Geometry: final body of the model. Coordinates: model frame, mm. A direction names the side the tool comes from. Give positions to 0.01 mm unless a question says otherwise; leave off trailing zeros. Write each loop counter-clockwise with the first axis right and the second up, starting at its lowest first coordinate (ties: lowest second). Pieces come first, ordered by that corner, then holes. Notation, with made-up numbers: M 0.5,13.5 L 36.5,13.5 A17 cw 36.5,24.5 Z; hole C 80.25,-12 d9. An arc over 180 degrees is marked long. Use one line per item in the form item = value. Start each with the question number.
Item 1: Material intervals for line 1 along Y through (x, z) = (37, 4.6); line 2 along X through (y, z) = (-3, 4.8); line 3 along X through (y, z) = (27, 3.95), sorted ascending. Write a range as from..to.
Item 2: Access query for faces 4 (the flat face through (-24.4, 4.5, 4.6)), 5 (the flat face through (63, 1, 5.08)). Directions: +Z, -Z, +X, -X, +Y, -Y. A direction counts if a zero-diameter tool reaches every point of the face in a straight line with its end or side. Return the directions, or none.
Item 3: Contact query for flat-ended pins moving along their axis: P1, Ø2, axis at x = 31, z = 4.5, coming from the -Y side; P2, Ø0.8, axis at x = 57, y = 29.5, coming from the -Z side; P3, Ø2, axis at x = 91.5, y = 29.5, coming from the +Z side; P4, Ø1.4, axis at x = 28, z = 1.5, coming from the +Y side. Output: stop coordinate, or through.
Item 4: Pull-direction query (X, two-part tool) for faces 1 (the flat face through (-32.034, 0, 3)), 2 (the flat face through (162.276, 0, 2)), 3 (the flat face through (-24.532, -4.383, 4.579)); classes: released by +X, released by -X, zero draft, split by the parting line, or undercut.
Item 5: Section query A-A on x = 20. Return loops of the section in (y, z).
Item 6: Section query B-B on x = -11. Return loops of the section in (y, z).
from build123d import *

# Parameters (mm, degrees)
F0_W     = 194.31
F0_H     = 54.864
F1_DEPTH = 5.08
F3_DEPTH = 194.31
F4_R     = 1.27
F6_DEPTH = 1.016


with BuildPart() as f1:
    # F0 (on Top) → F1 (new body)
    with BuildSketch(Plane.XY):
        with Locations((65.120992, 0.720159)):
            Rectangle(F0_W, F0_H)
    extrude(amount=F1_DEPTH)

    # F2 (on face) → F3 (join, through all)
    with BuildSketch(Plane(origin=(-32.034008, 0, 0), x_dir=(0, -1, 0), z_dir=(-1, 0, 0))):
        Polygon((-28.152159, 1.778), (-28.152159, 3.302), (-30.692159, 3.302), (-30.692159, 2.54), (-30.692159, 1.778), align=None)
        Polygon((29.251841, 3.302), (26.711841, 3.302), (26.711841, 1.778), (29.251841, 1.778), (29.251841, 2.54), align=None)
    extrude(amount=-F3_DEPTH)

    # F4
    f4_edges = [f1.edges().sort_by_distance(p)[0] for p in [
        (162.275992, 0.720159, 5.08),
    ]]
    fillet(f4_edges, radius=F4_R)

    # F5 (on face) → F6 (cut)
    with BuildSketch(Plane.XY.offset(5.08)):
        Polygon((-4.237764, -5.08), (-4.237764, 0), (-4.237764, 5.08), (-19.477764, 5.08), (-19.477764, 8.89), (-29.445775, 0), (-19.477764, -8.89), (-19.477764, -5.08), align=None)
    extrude(amount=-F6_DEPTH, mode=Mode.SUBTRACT)


solid = f1.part
Answer sheet:
q1.line_1 = -26.71..28.15
q1.line_2 = -32.03..-26.08, -4.24..161.8
q1.line_3 = -32.03..162.27
q2.face_4 = +Z
q2.face_5 = +Z, +X, -X, +Y, -Y
q3.P1 = -26.71
q3.P2 = 1.78
q3.P3 = 3.3
q3.P4 = 30.69
q4.face_1 = released by -X
q4.face_2 = released by +X
q4.face_3 = undercut
q5.outline = M -29.25,1.78 L -26.71,1.78 L -26.71,0 L 28.15,0 L 28.15,1.78 L 30.69,1.78 L 30.69,3.3 L 28.15,3.3 L 28.15,5.08 L -26.71,5.08 L -26.71,3.3 L -29.25,3.3 Z
q6.outline = M -29.25,1.78 L -26.71,1.78 L -26.71,0 L 28.15,0 L 28.15,1.78 L 30.69,1.78 L 30.69,3.3 L 28.15,3.3 L 28.15,5.08 L 5.08,5.08 L 5.08,4.06 L -5.08,4.06 L -5.08,5.08 L -26.71,5.08 L -26.71,3.3 L -29.25,3.3 Z
